from build123d import *

# Parameters (mm, degrees)
F0_R      = 18
F0_R_2    = 3
F0_W      = 3
F0_H      = 29
F0_H_2    = 15
F0_R_3    = 12.5
F1_DEPTH  = 20
F2_DEPTH  = 25
F4_DEPTH  = 25
F5_W      = 22
F5_H      = 19
F6_DEPTH  = 25
F8_DEPTH  = 25
F9_R      = 3
F10_DEPTH = 25


with BuildPart() as f1:
    # F0 (on Front) → F1 (new body)
    with BuildSketch(Plane.XZ):
        Polygon((60, 50), (60, 0), (155, 0), (155, 90), (63, 90), (63, 75), (60, 75), align=None)
        Polygon((1, 75), (60, 75), (60, 90), (60, 119), (1, 119), align=None)
        with Locations((32, 98)):
            Circle(F0_R, mode=Mode.SUBTRACT)
        Polygon((-5, 50), (60, 50), (60, 75), (1, 75), (1, 119), (60, 119), (60, 120), (-5, 120), align=None)
        with Locations((32, 71)):
            Circle(F0_R_2, mode=Mode.SUBTRACT)
        with Locations((50, 71)):
            Circle(F0_R_2, mode=Mode.SUBTRACT)
        Polygon((63, 90), (155, 90), (155, 150), (-5, 150), (-5, 120), (60, 120), (60, 119), (63, 119), align=None)
        with Locations((32, 125)):
            Circle(F0_R_2, mode=Mode.SUBTRACT)
        with Locations((50, 125)):
            Circle(F0_R_2, mode=Mode.SUBTRACT)
        with Locations((61.5, 104.5)):
            Rectangle(F0_W, F0_H)
        with Locations((61.5, 82.5)):
            Rectangle(F0_W, F0_H_2)
        with Locations((32, 98)):
            Circle(F0_R_3)
        with Locations((32, 98)):
            Circle(F0_R)
        with Locations((32, 98)):
            Circle(F0_R_3, mode=Mode.SUBTRACT)
        Polygon((-5, 50), (60, 0), (60, 50), align=None)
    extrude(amount=F1_DEPTH)

    # F0 (on Front) → F2 (cut)
    with BuildSketch(Plane.XZ):
        with Locations((32, 98)):
            Circle(F0_R_3)
    extrude(amount=F2_DEPTH, mode=Mode.SUBTRACT)

    # F3 (on face) → F4 (cut)
    with BuildSketch(Plane.XZ.offset(20)):
        with BuildLine():
            Line((65, 0), (155, 0))
            Line((155, 0), (155, 90))
            Line((155, 90), (70, 90))
            ThreePointArc((70, 90), (66.464466, 88.535534), (65, 85))
            Line((65, 85), (65, 0))
        make_face()
    extrude(amount=-F4_DEPTH, mode=Mode.SUBTRACT)

    # F5 (on face) → F6 (cut)
    with BuildSketch(Plane(origin=(0, 0, 0), x_dir=(-1, 0, 0), z_dir=(0, 1, 0))):
        with Locations((-87, 99.5)):
            Rectangle(F5_W, F5_H)
    extrude(amount=-F6_DEPTH, mode=Mode.SUBTRACT)

    # F7 (on face) → F8 (cut)
    with BuildSketch(Plane.XZ.offset(20)):
        with BuildLine():
            Line((155, 150), (60, 150))
            Line((60, 150), (60, 90))
            Line((60, 90), (65, 90))
            Line((65, 90), (65, 85))
            ThreePointArc((65, 85), (66.464466, 88.535534), (70, 90))
            Line((70, 90), (76, 90))
            Line((76, 90), (76, 109))
            Line((76, 109), (98, 109))
            Line((98, 109), (98, 90))
            Line((98, 90), (155, 90))
            Line((155, 90), (155, 150))
        make_face()
    extrude(amount=-F8_DEPTH, mode=Mode.SUBTRACT)

    # F9 (on face) → F10 (cut)
    with BuildSketch(Plane.XZ.offset(20)):
        with Locations((5, 140)):
            Circle(F9_R)
        with Locations((50, 140)):
            Circle(F9_R)
        with Locations((5, 60)):
            Circle(F9_R)
        with Locations((55, 20)):
            Circle(F9_R)
    extrude(amount=-F10_DEPTH, mode=Mode.SUBTRACT)


solid = f1.part
Check sheet for the modelled part. Datum: model origin and axes. Units: mm. A direction names the side the tool comes from. Coordinates: 2 decimals unless noted, no trailing zeros. Write each loop counter-clockwise with the first axis right and the second up, starting at its lowest first coordinate (ties: lowest second). Pieces come first, ordered by that corner, then holes.
Item 1: Depth check by flat-ended pin: pin 1 Ø1 at (y, z) = (-6.5, 45.5) entering from -X; pin 2 Ø10 at (x, y) = (3, -17.5) entering from -Z. Enter the tip coordinate at first touch or a pass-through.
Numbers:
pin 1: stops at x = 0.2
pin 2: stops at z = 40
Item 2: Access from +Z, -Z, +X, -X, +Y, -Y to the whole of each face (thin tool, end or side, straight path). Record for faces 1 (the face through (62, -10, 90)), 2 (the face through (52, -10, 20)).
Numbers:
face 1: +Z, +X, +Y, -Y
face 2: +Y, -Y
Item 3: Cross-section at A-A on z = 60. Record the boundary of the cut face in (x, y), then the cut area to 3 significant figures.
Numbers:
outline: (-5, -20) - (2, -20) - (2, 0) - (-5, 0) - close; (8, -20) - (65, -20) - (65, 0) - (8, 0) - close
area: 1,280 mm2
Item 4: Cross-section at D-D on x = 5. Record the boundary of the cut face in (y, z).
Numbers:
outline: (-20, 42.31) - (0, 42.31) - (0, 57) - (-20, 57) - close; (-20, 63) - (0, 63) - (0, 137) - (-20, 137) - close; (-20, 143) - (0, 143) - (0, 150) - (-20, 150) - close
Item 5: Cross-section at C-C on y = -13. Count the separate pieces of the cut face and the enclosed holes in it, then the cut area to 3 significant figures.
Numbers:
separate pieces: 1
enclosed holes: 9
area: 7,860 mm2
Item 6: Cross-section at B-B on z = 140. Record the boundary of the cut face in (x, y).
Numbers:
outline: (-5, -20) - (2, -20) - (2, 0) - (-5, 0) - close; (8, -20) - (47, -20) - (47, 0) - (8, 0) - close; (53, -20) - (60, -20) - (60, 0) - (53, 0) - close
Item 7: Scan lines: probe 1 along X at (y, z) = (-14.5, 140); probe 2 along Z at (x, y) = (32, -12); probe 3 along Z at (x, y) = (50, -4). Record each from-to range of solid material in increasing order.
Numbers:
probe 1: x = -5 to 2, 8 to 47, 53 to 60
probe 2: z = 21.54 to 68, 74 to 85.5, 110.5 to 122, 128 to 150
probe 3: z = 7.69 to 68, 74 to 122, 128 to 137, 143 to 150
Item 8: Mould release check, pull along X, two halves, no side actions. Record for faces 3 (the face through (30, -20, 76)), 4 (the face through (-5, -10, 101)), 5 (the face through (29.79, -9.86, 127.03)): released by +X, released by -X, zero draft, split by the parting line, or undercut.
Numbers:
face 3: zero draft
face 4: released by -X
face 5: undercut
